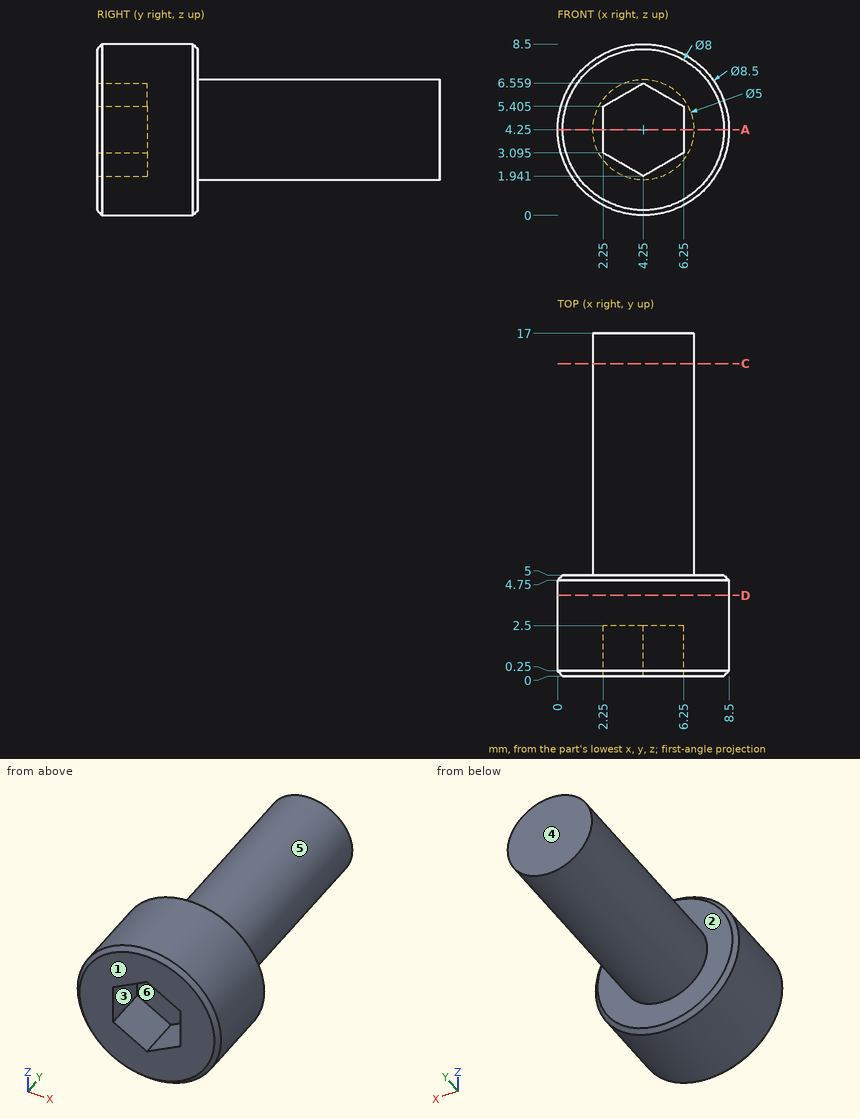
Input: dimensioned drawing with shaded views. Units: mm. Origin: part minimum x, y, z. A direction names the side the tool comes from. Give positions to 0.01 mm unless a question says otherwise; leave off trailing zeros. Write each loop counter-clockwise with the first axis right and the second up, starting at its lowest first coordinate (ties: lowest second). Pieces come first, ordered by that corner, then holes. Notation, with made-up numbers: M -24.5,52.5 L 25.5,52.5 A20 cw 25.5,77.5 Z; hole C 28,50 d5. An arc over 180 degrees is marked long. Write item = value, one per line. Start each with the question number.
1) First-contact query: pin 1 Ø2 at (x, y) = (6.5, 5) entering from +Z; pin 2 Ø1 at (x, y) = (6.5, 12.5) entering from +Z (1 decimal); pin 3 Ø2 at (x, z) = (4, 4.5) entering from -Y. Flat tips, straight axial feed; report the tip coordinate or a pass-through.
2) Draft query along X for the marked faces 4, 5 and 6. Return one class per face: +X half, -X half, draft (parallel to the pull), parting line (faces both ways), or undercut.
3) Cut plane C-C on y = 15.5. Return the cut outline in (x, z), then the cut area to 3 significant figures.
4) Material intervals for line 1 along Y through (x, z) = (3.75, 4.25); line 2 along X through (y, z) = (1.5, 4.75); line 3 along Y through (x, z) = (1.5, 4), sorted ascending. Write a range as [from, to].
5) Cut plane A-A on z = 4.25. Return the cut outline in (x, y).
6) Reachability of the marked faces 1, 2 and 3 from +Z, -Z, +X, -X, +Y, -Y: full face, straight path, thin tool, end or side. Return the list, or none.
7) Cut plane D-D on y = 4. Return the cut outline in (x, z).
Solved:
q1.pin_1 = 8.3
q1.pin_2 = 6
q1.pin_3 = 2.5
q2.face_4 = draft
q2.face_5 = parting line
q2.face_6 = undercut
q3.outline = C 4.25,4.25 d5
q3.area = 19.6 mm2
q4.line_1 = [2.5, 17]
q4.line_2 = [0.03, 2.25], [6.25, 8.47]
q4.line_3 = [0, 5]
q5.outline = M 0,0.25 L 0.25,0 L 2.25,0 L 2.25,2.5 L 6.25,2.5 L 6.25,0 L 8.25,0 L 8.5,0.25 L 8.5,4.75 L 8.25,5 L 6.75,5 L 6.75,17 L 1.75,17 L 1.75,5 L 0.25,5 L 0,4.75 Z
q6.face_1 = +Z, -Z, +X, -X, -Y
q6.face_2 = +Y
q6.face_3 = -Y
q7.outline = C 4.25,4.25 d8.5
